Part model, mm, in its own coordinate system. Face numbers are marked on the shaded views. A direction names the side the tool comes from. Round coordinates to 2 decimals unless told otherwise and drop trailing zeros. Order: outer loops, then holes, each group sorted by start corner. A loop starts at its lowest first (then second) coordinate and runs counter-clockwise, first axis right, second up. Notation, with made-up numbers: (-23.5, 72) - (-6.5, 72) arc R13 ccw to (-6.5, 90) - close; hole circle Ø9 at (47.5, -0.75). An arc over 180 degrees is marked (long way). Return JSON: item names as keys, results as strings. Group by question number.
Item 1: Drop flat-ended pins along their axis: pin 1 (4 mm diameter, centred on x = 5.5, y = 4, fed in from -Z); pin 2 (3 mm diameter, centred on x = 1, z = 3.5, fed in from -Y); pin 3 (5 mm diameter, centred on x = 3, z = 15, fed in from +Y). Give the stop position or say it passes through.
Item 2: Saw through at A-A on z = 11.43. List the corners of the cut face in (x, y), and give its area (3 significant figures).
Item 3: Saw through at B-B on x = 8.75. List the corners of the cut face in (y, z), and give its area (3 significant figures).
Item 4: Two-plate mould, pull along Y, no slides. Class the marked faces 1, 2 and 3: released by +Y, released by -Y, zero draft, split by the parting line, or undercut.
Item 5: Saw through at C-C on x = 4.75. List the corners of the cut face in (y, z).
Item 6: Probe probe 1 along Y at (x, z) = (5.5, 15.5); probe 2 along Z at (x, y) = (-5, 11). List the from-to ranges inside material, lowest first.
Item 7: Tool access for the marked faces 4 and 5: list every direction of +Z, -Z, +X, -X, +Y, -Y with a clear straight run to the whole face (end or side of a thin tool).
Item 8: Saw through at D-D on y = -3.25. List the corners of the cut face in (x, z).
```python
from build123d import *

# Parameters (mm, degrees)
SKETCH1_R               = 2.4892
BOSS_EXTRUDE1_DEPTH     = 6.35
BOSS_EXTRUDE2_START     = -6.35
BOSS_EXTRUDE2_DEPTH     = 19.05
BOSS_EXTRUDE2_START_2   = -6.555460136
BOSS_EXTRUDE2_2_DEPTH   = 19.460920272
BOSS_EXTRUDE2_START_3   = -10
BOSS_EXTRUDE2_3_DEPTH   = 3.65
CUT_EXTRUDE1_DEPTH      = 27.910448217
CUT_EXTRUDE1_DEPTH_BACK = 27.910448217
SKETCH3_W               = 2.179354936
SKETCH3_H               = 6.35
CUT_EXTRUDE2_DEPTH      = 31.98795935
CUT_EXTRUDE2_DEPTH_BACK = 31.98795935


with BuildPart() as part:
    # Sketch1 → Boss-Extrude1 (new body)
    with BuildSketch(Plane(origin=(0, 0, 0), x_dir=(1, 0, 0), z_dir=(0, 1, 0))):
        with BuildLine():
            Line((9.525, -17.889269346), (-0.578271622, -16.817120786))
            Line((-0.578271622, -16.817120786), (-6.35, 0))
            Line((-6.35, 0), (12.7, 0))
            Line((12.7, 0), (12.7, -6.35))
            ThreePointArc((12.7, -6.35), (15.186560179, -13.240601753), (9.525, -17.889269346))
        make_face()
        with Locations(Location((9.525, -11.43, 0), (0, 0, 270))):
            Circle(SKETCH1_R, mode=Mode.SUBTRACT)
    extrude(amount=BOSS_EXTRUDE1_DEPTH)

    # Boss-Extrude2: read off the stored shape, not the designer's step
    # Boss-Extrude2 outline → Boss-Extrude2 (add)
    with BuildSketch(Plane.YZ.offset(BOSS_EXTRUDE2_START)):
        with BuildLine():
            ThreePointArc((11.551615481, -6.35), (12.905510296, -4.996105185), (11.551615481, -3.642210371))
            Line((11.551615481, -3.642210371), (6.35, 0))
            Line((6.35, 0), (0, 0))
            Line((0, 0), (-5.201615481, -3.642210371))
            ThreePointArc((-5.201615481, -3.642210371), (-6.555510296, -4.996105185), (-5.201615481, -6.35))
            Line((-5.201615481, -6.35), (11.551615481, -6.35))
        make_face()
    extrude(amount=BOSS_EXTRUDE2_DEPTH)

    # Boss-Extrude2 2 outline → Boss-Extrude2 2 (add)
    with BuildSketch(Plane(origin=(0, 0, 0), x_dir=(1, 0, 0), z_dir=(0, 1, 0)).offset(BOSS_EXTRUDE2_START_2)):
        Polygon((-8.529354936, 6.35), (-6.35, 0), (-6.35, 6.35), align=None)
    extrude(amount=BOSS_EXTRUDE2_2_DEPTH)

    # Boss-Extrude2 3 outline → Boss-Extrude2 3 (cut)
    with BuildSketch(Plane.YZ.offset(BOSS_EXTRUDE2_START_3)):
        with BuildLine():
            Line((12.905460136, 0), (6.35, 0))
            Line((6.35, 0), (11.551615481, -3.642210371))
            ThreePointArc((11.551615481, -3.642210371), (12.504834401, -4.034645431), (12.905460136, -4.984450993))
            Line((12.905460136, -4.984450993), (12.905460136, 0))
        make_face()
        with BuildLine():
            ThreePointArc((12.905460136, -5.007759378), (12.504834401, -5.95756494), (11.551615481, -6.35))
            Line((11.551615481, -6.35), (12.905460136, -6.35))
            Line((12.905460136, -6.35), (12.905460136, -5.007759378))
        make_face()
        with BuildLine():
            Line((0, 0), (-6.555460136, 0))
            Line((-6.555460136, 0), (-6.555460136, -4.984450993))
            ThreePointArc((-6.555460136, -4.984450993), (-6.154834401, -4.034645431), (-5.201615481, -3.642210371))
            Line((-5.201615481, -3.642210371), (0, 0))
        make_face()
        with BuildLine():
            ThreePointArc((-5.201615481, -6.35), (-6.154834401, -5.95756494), (-6.555460136, -5.007759378))
            Line((-6.555460136, -5.007759378), (-6.555460136, -6.35))
            Line((-6.555460136, -6.35), (-5.201615481, -6.35))
        make_face()
    extrude(amount=BOSS_EXTRUDE2_3_DEPTH, mode=Mode.SUBTRACT)

    # Sketch3 → Cut-Extrude1 (cut, two sides: drawn at the far end of the back side and taken through both)
    with BuildSketch(Plane.XZ.offset(-CUT_EXTRUDE1_DEPTH_BACK)):
        with Locations((-7.439677468, -3.175)):
            Rectangle(SKETCH3_W, SKETCH3_H)
    extrude(amount=CUT_EXTRUDE1_DEPTH + CUT_EXTRUDE1_DEPTH_BACK, mode=Mode.SUBTRACT)

    # Sketch4 → Cut-Extrude2 (cut, two sides: drawn at the far end of the back side and taken through both)
    with BuildSketch(Plane.ZY.offset(6.35).offset(-CUT_EXTRUDE2_DEPTH_BACK)):
        with BuildLine():
            ThreePointArc((-5.588, -4.764550237), (-4.927202114, -5.833718802), (-4.266404229, -4.764550237))
            Line((-4.266404229, -4.764550237), (-0.930230237, 0))
            Line((-0.930230237, 0), (0, 0))
            Line((0, 0), (-3.642210371, -5.201615481))
            ThreePointArc((-3.642210371, -5.201615481), (-4.996105185, -6.555510296), (-6.35, -5.201615481))
            Line((-6.35, -5.201615481), (-6.35, 11.551615481))
            ThreePointArc((-6.35, 11.551615481), (-4.996105185, 12.905510296), (-3.642210371, 11.551615481))
            Line((-3.642210371, 11.551615481), (0, 6.35))
            Line((0, 6.35), (-0.930230237, 6.35))
            Line((-0.930230237, 6.35), (-4.266404229, 11.114550237))
            ThreePointArc((-4.266404229, 11.114550237), (-4.927202114, 12.183718802), (-5.588, 11.114550237))
            Line((-5.588, 11.114550237), (-5.588, -4.764550237))
        make_face()
    extrude(amount=CUT_EXTRUDE2_DEPTH + CUT_EXTRUDE2_DEPTH_BACK, mode=Mode.SUBTRACT)


solid = part.part
```
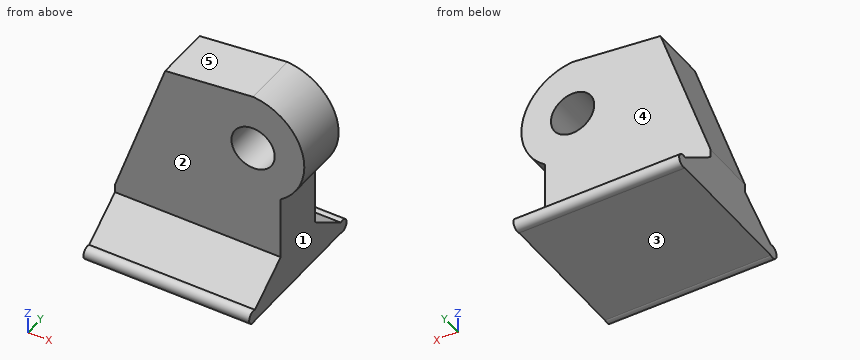
Filled in:
{
 "1": {"pin 1": "stops at z = -5.59", "pin 2": "stops at y = 0", "pin 3": "stops at y = 6.35"},
 "2": {"outline": "(-2.43, 0) - (7.04, 0) - (7.04, 6.35) - (-2.43, 6.35) - close; (12.01, 0) - (15.41, 0) - (15.41, 6.35) - (12.01, 6.35) - close", "area": "81.7 mm^2"},
 "3": {"outline": "(-4.76, -5.59) - (11.11, -5.59) arc R0.74 ccw (long way) to (11.11, -4.27) - (6.35, -0.93) - (6.35, 9.06) - (0, 9.06) - (0, -0.93) - (-4.76, -4.27) arc R0.74 ccw (long way) to start; (0, 13.8) - (6.35, 13.8) - (6.35, 17.81) - (0, 17.81) - close", "area": "150 mm^2"},
 "4": {"face 1": "zero draft", "face 2": "released by -Y", "face 3": "undercut"},
 "5": {"outline": "(-4.76, -5.59) - (11.11, -5.59) arc R0.74 ccw (long way) to (11.11, -4.27) - (6.35, -0.93) - (6.35, 17.38) - (0, 17.38) - (0, -0.93) - (-4.76, -4.27) arc R0.74 ccw (long way) to start"},
 "6": {"probe 1": "y = 0 to 6.35", "probe 2": "z = -5.59 to -4.19"},
 "7": {"face 4": "+Z, +X, -X, +Y", "face 5": "+Z, -X, +Y, -Y"},
 "8": {"outline": "(-6.35, -5.59) - (12.7, -5.59) - (12.7, -3.21) - (-6.35, -3.21) - close"}
}
